Geometry: final body of the model. Coordinates: model frame, mm. Round coordinates to 2 decimals unless told otherwise and drop trailing zeros. Order: outer loops, then holes, each group sorted by start corner. A loop starts at its lowest first (then second) coordinate and runs counter-clockwise, first axis right, second up. Notation, with made-up numbers: M -7.75,74 L 19.25,74 A19 ccw 19.25,91 Z; hole C 72.25,45.25 d2. An arc over 180 degrees is marked long. Return JSON: item names as keys, results as strings. Group by question number.
Q1. Cut plane A-A on x = 0. Output: boundary loops of the cut face in (y, z).
Q2. Cut plane B-B on z = 89. Output: boundary loops of the cut face in (x, y), and give its area (3 significant figures).
Q3. Ray query, probe 1 along Z at (x, y) = (0, 2.2); probe 2 along Z at (x, y) = (30, 0.75); probe 3 along Z at (x, y) = (28, 2.4). Return the intervals inside material, ascending.
Q4. Cut plane C-C on y = 1.3. Output: boundary loops of the cut face in (x, z), and give its area (3 significant figures).
Q5. Cut plane D-D on x = -27.5. Output: boundary loops of the cut face in (y, z).
```python
from build123d import *

# Parameters (mm, degrees)
F0_R     = 2
F1_DEPTH = 3
F2_SIZE2 = 12
F2_SIZE  = 15


with BuildPart() as f1:
    # F0 (on Front) → F1 (new body)
    with BuildSketch(Plane.XZ):
        Polygon((-35, 0), (0, 0), (35, 0), (35, 97), (0, 97), (-35, 97), align=None)
        with Locations((0, 89)):
            Circle(F0_R, mode=Mode.SUBTRACT)
    extrude(amount=-F1_DEPTH)

    # F2
    f2_edges = [f1.edges().sort_by_distance(p)[0] for p in [
        (-35, 1.5, 97),
        (35, 1.5, 97),
    ]]
    f2_side = f1.faces().sort_by_distance((0, 1.5, 97))[0]
    chamfer(f2_edges, length=F2_SIZE, length2=F2_SIZE2, reference=f2_side)


solid = f1.part
```
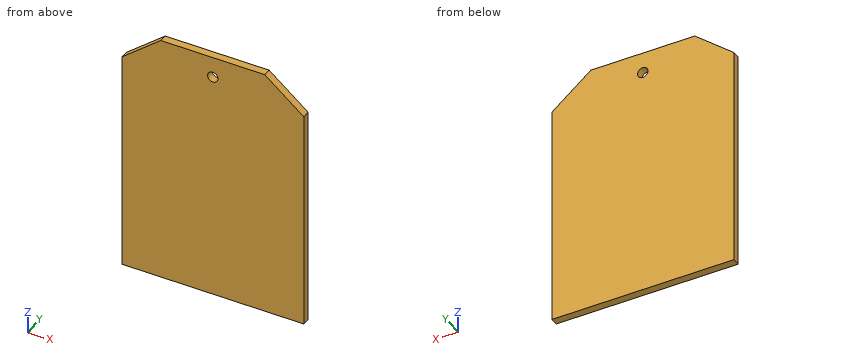
Result sheet:
{
 "1": {"outline": "M 0,0 L 3,0 L 3,87 L 0,87 Z; M 0,91 L 3,91 L 3,97 L 0,97 Z"},
 "2": {"outline": "M -30,0 L -2,0 L -2,3 L -30,3 Z; M 2,0 L 30,0 L 30,3 L 2,3 Z", "area": "168 mm²"},
 "3": {"probe 1": "z = 0 to 87, 91 to 97", "probe 2": "z = 0 to 89", "probe 3": "z = 0 to 90.6"},
 "4": {"outline": "M -35,0 L 35,0 L 35,85 L 20,97 L -20,97 L -35,85 Z; hole C 0,89 d4", "area": "6,600 mm²"},
 "5": {"outline": "M 0,0 L 3,0 L 3,91 L 0,91 Z"}
}
